Read the model definition and answer for the solid it produces. Units are mm, in the model's axes. A direction names the side the tool comes from. Coordinates: 2 decimals unless noted, no trailing zeros. Order: outer loops, then holes, each group sorted by start corner. A loop starts at its lowest first (then second) coordinate and runs counter-clockwise, first axis right, second up. Notation, with made-up numbers: (80.25, 28) -> (103.25, 28) arc R16 cw to (103.25, 59) -> close; hole circle Ø6 at (-21, 18). An arc over 180 degrees is marked (long way). Use CSV: the item, a comma, the result in double quotes.
```python
from build123d import *

# Parameters (mm, degrees)
BOSS_EXTRUDE1_DEPTH   = 700
BOSS_EXTRUDE1_2_DEPTH = 700
BOSS_EXTRUDE2_DEPTH   = 200
SKETCH1_4_W           = 400
SKETCH1_4_H           = 150
BOSS_EXTRUDE3_DEPTH   = 800
SKETCH1_5_W           = 500
SKETCH1_5_H           = 80
BOSS_EXTRUDE4_DEPTH   = 150
SKETCH1_6_W           = 500
SKETCH1_6_H           = 80
BOSS_EXTRUDE5_DEPTH   = 100
SKETCH1_7_W           = 250
SKETCH1_7_H           = 80
BOSS_EXTRUDE6_DEPTH   = 50


with BuildPart() as part:
    # Sketch1 → Boss-Extrude1 (new body)
    with BuildSketch(Plane(origin=(0, 0, 0), x_dir=(1, 0, 0), z_dir=(0, 1, 0))):
        Polygon((350, 240), (500, 240), (500, 540), (200, 540), (200, 390), (350, 390), align=None)
    extrude(amount=BOSS_EXTRUDE1_DEPTH)



with BuildPart() as body_2:
    # Sketch1 → Boss-Extrude1 2 (new body)
    with BuildSketch(Plane(origin=(0, 0, 0), x_dir=(1, 0, 0), z_dir=(0, 1, 0))):
        Polygon((-500, 540), (-500, 240), (-350, 240), (-350, 390), (-200, 390), (-200, 540), align=None)
    extrude(amount=BOSS_EXTRUDE1_2_DEPTH)


with BuildPart() as part_1:
    add(part.part)

    add(body_2.part)  # Boss-Extrude2 merges body 2
    # Sketch1_3 → Boss-Extrude2 (add)
    with BuildSketch(Plane(origin=(0, 0, 0), x_dir=(1, 0, 0), z_dir=(0, 1, 0))):
        Polygon((-500, 240), (-500, 0), (-250, 0), (-250, 80), (-250, 160), (-250, 240), (250, 240), (250, 160), (250, 80), (250, 0), (500, 0), (500, 240), (350, 240), (350, 390), (200, 390), (-200, 390), (-350, 390), (-350, 240), align=None)
    extrude(amount=BOSS_EXTRUDE2_DEPTH)

    # Sketch1_4 → Boss-Extrude3 (add)
    with BuildSketch(Plane(origin=(0, 0, 0), x_dir=(1, 0, 0), z_dir=(0, 1, 0))):
        with Locations((0, 465)):
            Rectangle(SKETCH1_4_W, SKETCH1_4_H)
    extrude(amount=BOSS_EXTRUDE3_DEPTH)

    # Sketch1_5 → Boss-Extrude4 (add)
    with BuildSketch(Plane(origin=(0, 0, 0), x_dir=(1, 0, 0), z_dir=(0, 1, 0))):
        with Locations((0, 200)):
            Rectangle(SKETCH1_5_W, SKETCH1_5_H)
    extrude(amount=BOSS_EXTRUDE4_DEPTH)

    # Sketch1_6 → Boss-Extrude5 (add)
    with BuildSketch(Plane(origin=(0, 0, 0), x_dir=(1, 0, 0), z_dir=(0, 1, 0))):
        with Locations((0, 120)):
            Rectangle(SKETCH1_6_W, SKETCH1_6_H)
    extrude(amount=BOSS_EXTRUDE5_DEPTH)

    # Sketch1_7 → Boss-Extrude6 (add)
    with BuildSketch(Plane(origin=(0, 0, 0), x_dir=(1, 0, 0), z_dir=(0, 1, 0))):
        with Locations((125, 40)):
            Rectangle(SKETCH1_7_W, SKETCH1_7_H)
        with Locations((-125, 40)):
            Rectangle(SKETCH1_7_W, SKETCH1_7_H)
    extrude(amount=BOSS_EXTRUDE6_DEPTH)


solid = part_1.part
```
Item 1: Find section C-C, the plane z = -110. Give the vertices of the cut face in (x, y), then the cut area to 3 significant figures.
Return value:
outline,"(-500, 0) -> (500, 0) -> (500, 200) -> (250, 200) -> (250, 100) -> (-250, 100) -> (-250, 200) -> (-500, 200) -> close"
area,"150,000 mm^2"
Item 2: Find section A-A, the plane x = 231.5. Give the vertices of the cut face in (y, z).
Return value:
outline,"(0, -540) -> (700, -540) -> (700, -390) -> (200, -390) -> (200, -240) -> (150, -240) -> (150, -160) -> (100, -160) -> (100, -80) -> (50, -80) -> (50, 0) -> (0, 0) -> close"
Item 3: A tool of negligible diameter and unlimited length cuts with its end or side. For faces 4 (the flat face through (-350, 446, -314)), 5 (the flat face through (-500, 267, -334)), 6 (the flat face through (381, 700, -425)), 7 (the flat face through (-385, 700, -425)), 8 (the flat face through (424, 446, -240)), from which of +Z, -Z, +X, -X, +Y, -Y can it reach the whole face along a straight path? Write none if from no direction.
Return value:
face 4,"+Z, +Y"
face 5,"+Z, -Z, -X, +Y, -Y"
face 6,"+Z, -Z, +X, +Y"
face 7,"+Z, -Z, -X, +Y"
face 8,"+Z, +X, -X, +Y"
Item 4: Find section B-B, the plane y = 510.5. Give the vertices of the cut face in (x, z), then the cut area to 3 significant figures.
Return value:
outline,"(-500, -540) -> (500, -540) -> (500, -240) -> (350, -240) -> (350, -390) -> (-350, -390) -> (-350, -240) -> (-500, -240) -> close"
area,"195,000 mm^2"
Item 5: Straight lines are drawn through the part: line 1 along X through (y, z) = (514, -326); line 2 along X through (y, z) = (141.5, -51); line 3 along Z through (x, y) = (433, 258). For each, find the intervals that lie inside material, in ascending order.
Return value:
line 1,"x = -500 to -350, 350 to 500"
line 2,"x = -500 to -250, 250 to 500"
line 3,"z = -540 to -240"
Item 6: Each of these flat-tipped pins is pushed along its axis until it touches: P1, Ø15, axis at x = 1, y = 118.5, coming from the +Z side; P2, Ø2, axis at x = -281.5, z = -70, coming from the +Y side; P3, Ø8, axis at x = 369, y = 609, coming from the +Z side; P4, Ø1, axis at x = -195.5, z = -75.5, coming from the -Y side. Where does it stop, or does it pass through?
Return value:
P1,"stops at z = -160"
P2,"stops at y = 200"
P3,"stops at z = -240"
P4,"stops at y = 0"
Item 7: The mould has two halves that part along X. Classify faces 1 (the flat face through (-250, 141, -92)), 2 (the flat face through (500, 267, -326)), 3 (the flat face through (-200, 749, -464)): +X half, -X half, draft (parallel to the pull), parting line (faces both ways), or undercut.
Return value:
face 1,"undercut"
face 2,"+X half"
face 3,"-X half"
Item 8: Find section D-D, the plane x = -65. Give the vertices of the cut face in (y, z).
Return value:
outline,"(0, -540) -> (800, -540) -> (800, -390) -> (200, -390) -> (200, -240) -> (150, -240) -> (150, -160) -> (100, -160) -> (100, -80) -> (50, -80) -> (50, 0) -> (0, 0) -> close"
